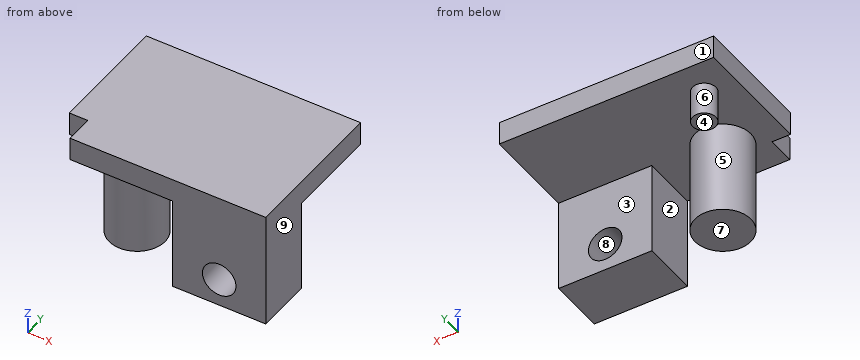
```python
from build123d import *

# Parameters (mm, degrees)
BOSS_EXTRUDE1_DEPTH = 2.5
SKETCH2_R           = 1.25
BOSS_EXTRUDE2_DEPTH = 3.5
SKETCH3_R           = 3
BOSS_EXTRUDE3_DEPTH = 10
SKETCH4_W           = 10
SKETCH4_H           = 6
BOSS_EXTRUDE4_DEPTH = 10
SKETCH5_R           = 1.8
CUT_EXTRUDE1_DEPTH  = 7
BOSS_EXTRUDE5_DEPTH = 2.5
SKETCH8_W           = 7
SKETCH8_H           = 30
CUT_EXTRUDE2_DEPTH  = 10
SKETCH9_W           = 15.6
SKETCH9_H           = 14
CUT_EXTRUDE3_DEPTH  = 10
SKETCH10_W          = 2
SKETCH10_H          = 16
CUT_EXTRUDE4_DEPTH  = 10
SKETCH11_R          = 1.25
BOSS_EXTRUDE6_DEPTH = 3.5
SKETCH12_W          = 2
SKETCH12_H          = 3
CUT_EXTRUDE5_DEPTH  = 10


with BuildPart() as part:
    # Sketch1 → Boss-Extrude1 (new body)
    with BuildSketch(Plane.XY):
        Polygon((-47.040141431, -25.701123128), (-19.040141431, -25.701123128), (-19.040141431, 4.298876872), (-29.040141431, 4.298876872), (-47.040141431, -15.701123128), align=None)
    extrude(amount=BOSS_EXTRUDE1_DEPTH)

    # Sketch2 → Boss-Extrude2 (add)
    with BuildSketch(Plane(origin=(0, 0, 0), x_dir=(-1, 0, 0), z_dir=(0, 0, -1))):
        with Locations((23.040141431, -0.081123128)):
            Circle(SKETCH2_R)
    extrude(amount=BOSS_EXTRUDE2_DEPTH)

    # Sketch3 → Boss-Extrude3 (add)
    with BuildSketch(Plane(origin=(0, 0, 0), x_dir=(-1, 0, 0), z_dir=(0, 0, -1))):
        with Locations((43.040141431, -20.701123128)):
            Circle(SKETCH3_R)
    extrude(amount=BOSS_EXTRUDE3_DEPTH)

    # Sketch4 → Boss-Extrude4 (add)
    with BuildSketch(Plane(origin=(0, 0, 0), x_dir=(-1, 0, 0), z_dir=(0, 0, -1))):
        with Locations((31.040141431, -22.701123128)):
            Rectangle(SKETCH4_W, SKETCH4_H)
    extrude(amount=BOSS_EXTRUDE4_DEPTH)

    # Sketch5 → Cut-Extrude1 (cut, through all)
    with BuildSketch(Plane(origin=(0, -19.701123128, 0), x_dir=(1, 0, 0), z_dir=(0, 1, 0))):
        with Locations((-31.040141431, 7)):
            Circle(SKETCH5_R)
    extrude(amount=-CUT_EXTRUDE1_DEPTH, mode=Mode.SUBTRACT)

    # Sketch6 → Boss-Extrude5 (add)
    with BuildSketch(Plane(origin=(0, 0, 0), x_dir=(-1, 0, 0), z_dir=(0, 0, -1))):
        Polygon((47.040141431, -25.701123128), (51.040141431, -25.701123128), (51.040141431, -9.701123128), (41.640141431, -9.701123128), (47.040141431, -15.701123128), align=None)
    extrude(amount=-BOSS_EXTRUDE5_DEPTH)

    # Sketch8 → Cut-Extrude2 (cut)
    with BuildSketch(Plane(origin=(0, 0, -3.5), x_dir=(-1, 0, 0), z_dir=(0, 0, -1))):
        with Locations((22.540141431, -10.701123128)):
            Rectangle(SKETCH8_W, SKETCH8_H)
    extrude(amount=-CUT_EXTRUDE2_DEPTH, mode=Mode.SUBTRACT)

    # Sketch9 → Cut-Extrude3 (cut)
    with BuildSketch(Plane(origin=(0, 0, 0), x_dir=(-1, 0, 0), z_dir=(0, 0, -1))):
        with Locations((33.840141431, -2.701123128)):
            Rectangle(SKETCH9_W, SKETCH9_H)
    extrude(amount=-CUT_EXTRUDE3_DEPTH, mode=Mode.SUBTRACT)

    # Sketch10 → Cut-Extrude4 (cut)
    with BuildSketch(Plane(origin=(0, 0, 0), x_dir=(-1, 0, 0), z_dir=(0, 0, -1))):
        with Locations((50.040141431, -17.701123128)):
            Rectangle(SKETCH10_W, SKETCH10_H)
    extrude(amount=-CUT_EXTRUDE4_DEPTH, mode=Mode.SUBTRACT)

    # Sketch11 → Boss-Extrude6 (add)
    with BuildSketch(Plane(origin=(0, 0, 0), x_dir=(-1, 0, 0), z_dir=(0, 0, -1))):
        with Locations((45.680141431, -13.401123128)):
            Circle(SKETCH11_R)
    extrude(amount=BOSS_EXTRUDE6_DEPTH)

    # Sketch12 → Cut-Extrude5 (cut)
    with BuildSketch(Plane(origin=(0, 0, 0), x_dir=(-1, 0, 0), z_dir=(0, 0, -1))):
        with Locations((48.040141431, -24.201123128)):
            Rectangle(SKETCH12_W, SKETCH12_H)
    extrude(amount=-CUT_EXTRUDE5_DEPTH, mode=Mode.SUBTRACT)


solid = part.part
```
Geometry check sheet. Reference: the model listing, model coordinates, mm. Face numbers are marked on the shaded views. A direction names the side the tool comes from. Give positions to 0.01 mm unless a question says otherwise; leave off trailing zeros. Write each loop counter-clockwise with the first axis right and the second up, starting at its lowest first coordinate (ties: lowest second). Pieces come first, ordered by that corner, then holes. Notation, with made-up numbers: (52, 35) -> (99, 35) arc R30 ccw to (99, 65) -> close; hole circle Ø10 at (30.25, -8.75). An arc over 180 degrees is marked (long way). Use one line per item in the form item = value.
Item 1: Scan lines: line 1 (X direction, y = -24.05, z = -7); line 2 (X direction, y = -21.6, z = -7); line 3 (X direction, y = -20.5, z = -3.25). Record each from-to range of solid material in increasing order.
Results list:
line_1 = -36.04 to -32.84, -29.24 to -26.04
line_2 = -45.9 to -40.18, -36.04 to -32.84, -29.24 to -26.04
line_3 = -46.03 to -40.05, -36.04 to -26.04
Item 2: Sectioned sample at B-B on y = -14.25. Enter the section's corners in (x, z).
Results list:
outline = (-49.04, 0) -> (-46.6, 0) -> (-46.6, -3.5) -> (-44.76, -3.5) -> (-44.76, 0) -> (-26.04, 0) -> (-26.04, 2.5) -> (-49.04, 2.5) -> close
Item 3: Sectioned sample at D-D on z = 0.5. Enter the section's corners in (x, y), plus the area to 3 significant figures.
Results list:
outline = (-49.04, -22.7) -> (-47.04, -22.7) -> (-47.04, -25.7) -> (-26.04, -25.7) -> (-26.04, -9.7) -> (-49.04, -9.7) -> close
area = 362 mm2
Item 4: Depth check by flat-ended pin: pin 1 Ø1 at (x, z) = (-48, 0.5) entering from -Y; pin 2 Ø3 at (x, y) = (-30, -15.5) entering from -Z; pin 3 Ø3 at (y, z) = (-24.5, 1.5) entering from -X. Enter the tip coordinate at first touch or a pass-through.
Results list:
pin_1 = -22.7
pin_2 = 0
pin_3 = -47.04
Item 5: Sectioned sample at A-A on z = -7. Enter the section's corners in (x, y).
Results list:
outline = circle Ø6 at (-43.04, -20.7); (-36.04, -25.7) -> (-32.84, -25.7) -> (-32.84, -19.7) -> (-36.04, -19.7) -> close; (-29.24, -25.7) -> (-26.04, -25.7) -> (-26.04, -19.7) -> (-29.24, -19.7) -> close
Item 6: Mould release check, pull along X, two halves, no side actions. Record for the marked faces 6, 7, 8 and 9: released by +X, released by -X, zero draft, split by the parting line, or undercut.
Results list:
face_6 = split by the parting line
face_7 = zero draft
face_8 = undercut
face_9 = released by +X
Item 7: Access from +Z, -Z, +X, -X, +Y, -Y to the whole of each face (thin tool, end or side, straight path). Record for the marked faces 1, 2, 3, 4 and 5.
Results list:
face_1 = +Z, -Z, +X, -X, +Y
face_2 = -Z, +Y, -Y
face_3 = -Z, +X, +Y
face_4 = -Z, +X, -X, +Y
face_5 = -Z
Item 8: Sectioned sample at C-C on x = -39. Enter the section's corners in (y, z).
Results list:
outline = (-25.7, 0) -> (-9.7, 0) -> (-9.7, 2.5) -> (-25.7, 2.5) -> close
